Here's how the part is built. I have some questions about the finished solid (model axes, mm). A direction names the side the tool comes from. Round coordinates to 2 decimals unless told otherwise and drop trailing zeros. Order: outer loops, then holes, each group sorted by start corner. A loop starts at its lowest first (then second) coordinate and runs counter-clockwise, first axis right, second up.
```python
from build123d import *

# Parameters (mm, degrees)
SKETCH1_W           = 116
SKETCH1_H           = 83
SKETCH1_W_2         = 70
SKETCH1_H_2         = 77
SKETCH1_W_3         = 35
BOSS_EXTRUDE1_DEPTH = 3
SKETCH2_W           = 70
SKETCH2_H           = 77
SKETCH2_W_2         = 35
BOSS_EXTRUDE2_DEPTH = 3
SKETCH6_R           = 1.75
CUT_EXTRUDE4_DEPTH  = 30
SKETCH8_W           = 20
SKETCH8_H           = 20
CUT_EXTRUDE6_DEPTH  = 10


with BuildPart() as part:
    # Sketch1 → Boss-Extrude1 (new body)
    with BuildSketch(Plane.XY):
        with Locations((-58, 41.5)):
            Rectangle(SKETCH1_W, SKETCH1_H)
        with Locations((-38, 41.5)):
            Rectangle(SKETCH1_W_2, SKETCH1_H_2, mode=Mode.SUBTRACT)
        with Locations((-95.5, 41.5)):
            Rectangle(SKETCH1_W_3, SKETCH1_H_2, mode=Mode.SUBTRACT)
    extrude(amount=BOSS_EXTRUDE1_DEPTH)

    # Sketch2 → Boss-Extrude2 (add)
    with BuildSketch(Plane(origin=(0, 0, 0), x_dir=(-1, 0, 0), z_dir=(0, 0, -1))):
        with Locations((38, 41.5)):
            Rectangle(SKETCH2_W, SKETCH2_H)
        with Locations((95.5, 41.5)):
            Rectangle(SKETCH2_W_2, SKETCH2_H)
    extrude(amount=-BOSS_EXTRUDE2_DEPTH)

    # Sketch6 → Cut-Extrude4 (cut)
    with BuildSketch(Plane.XY.offset(3)):
        with Locations((-75.5, 63)):
            Circle(SKETCH6_R)
        with Locations((-75.5, 20)):
            Circle(SKETCH6_R)
    extrude(amount=-CUT_EXTRUDE4_DEPTH, mode=Mode.SUBTRACT)

    # Sketch8 → Cut-Extrude6 (cut)
    with BuildSketch(Plane.XY.offset(3)):
        with Locations((-10, 60)):
            Rectangle(SKETCH8_W, SKETCH8_H)
    extrude(amount=-CUT_EXTRUDE6_DEPTH, mode=Mode.SUBTRACT)


solid = part.part
```
1. If we section it at C-C, the plane z = 0.7: Write out the boundary of the cut face in (x, y).
Evaluation:
outline: (-116, 0) - (0, 0) - (0, 50) - (-20, 50) - (-20, 70) - (0, 70) - (0, 83) - (-116, 83) - close; hole circle Ø3.5 at (-75.5, 20); hole circle Ø3.5 at (-75.5, 63)
2. If we mould it in two halves opening along X, with no side actions, what happens to faces 1 (the flat face through (0, 25, 1)), 2 (the flat face through (-116, 41, 1)), 3 (the cylindrical face through (-73.883, 62.33, 1.521))? For each: released by +X, released by -X, zero draft, split by the parting line, or undercut.
Evaluation:
face 1: released by +X
face 2: released by -X
face 3: undercut
3. If we section it at D-D, the plane x = -76: Write out the boundary of the cut face in (y, z).
Evaluation:
outline: (0, 0) - (18.32, 0) - (18.32, 3) - (0, 3) - close; (21.68, 0) - (61.32, 0) - (61.32, 3) - (21.68, 3) - close; (64.68, 0) - (83, 0) - (83, 3) - (64.68, 3) - close
4. If we section it at B-B, the plane x = -18.5: Write out the boundary of the cut face in (y, z).
Evaluation:
outline: (0, 0) - (50, 0) - (50, 3) - (0, 3) - close; (70, 0) - (83, 0) - (83, 3) - (70, 3) - close
5. I need wall thicknesses on probe 1 along Y at (x, z) = (-75.5, 0.7); probe 2 along Y at (x, z) = (-16, 0.5); probe 3 along X at (y, z) = (59.5, 0.2). Which ranges of each line are inside material? Lowest first, please.
Evaluation:
probe 1: y = 0 to 18.25, 21.75 to 61.25, 64.75 to 83
probe 2: y = 0 to 50, 70 to 83
probe 3: x = -116 to -20
6. On a 3-axis mill with a long thin cutter (end or side, diameter ignored), from which of +Z, -Z, +X, -X, +Y, -Y can I reach the whole of each face in a straight line? I mean faces 4 (the flat face through (-57, 42, 0)), 5 (the flat face through (-10, 70, 2)). Say none if no direction works.
Evaluation:
face 4: -Z, +X, -X, +Y, -Y
face 5: +Z, -Z, +X
7. I'm going to push flat-ended pins straight in: P1, Ø1.5, axis at x = -60, z = 1.5, coming from the -Y side; P2, Ø1.5, axis at y = 60, z = 1, coming from the +X side. Where does each tip first touch, or does it pass through?
Evaluation:
P1: stops at y = 0
P2: stops at x = -20
8. If we section it at A-A, the plane y = 63: Write out the boundary of the cut face in (x, z).
Evaluation:
outline: (-116, 0) - (-77.25, 0) - (-77.25, 3) - (-116, 3) - close; (-73.75, 0) - (-20, 0) - (-20, 3) - (-73.75, 3) - close
